```python
from build123d import *

# Parameters (mm, degrees)
EXTRUDE_THIN1_DEPTH = 342.9
CUT_EXTRUDE4_REACH  = 348.468
SKETCH2_R           = 2.667


with BuildPart() as part:
    # Sketch1 → Extrude-Thin1 (new, symmetric)
    with BuildSketch(Plane(origin=(0, 0, 0), x_dir=(0, 0, -1), z_dir=(1, 0, 0))):
        Polygon((-38.1, 0), (0, 0), (0, 38.1), (-6.35, 38.1), (-6.35, 6.35), (-38.1, 6.35), align=None)
    extrude(amount=EXTRUDE_THIN1_DEPTH, both=True)

    # Sketch2 → Cut-Extrude4 (cut, up to next)
    with BuildSketch(Plane(origin=(0, 6.35, 0), x_dir=(1, 0, 0), z_dir=(0, 1, 0)), mode=Mode.PRIVATE) as cut_extrude4_sk1:
        with Locations(Location((-336.55, -15.875, 0), (0, 0, 270))):
            Circle(SKETCH2_R)
    cut_extrude4_tool1 = extrude(cut_extrude4_sk1.sketch, amount=-CUT_EXTRUDE4_REACH, mode=Mode.PRIVATE) & part.part
    # Sketch2 → Cut-Extrude4 (cut, up to next)
    with BuildSketch(Plane(origin=(0, 6.35, 0), x_dir=(1, 0, 0), z_dir=(0, 1, 0)), mode=Mode.PRIVATE) as cut_extrude4_sk2:
        with Locations(Location((-273.05, -15.875, 0), (0, 0, 270))):
            Circle(SKETCH2_R)
    cut_extrude4_tool2 = extrude(cut_extrude4_sk2.sketch, amount=-CUT_EXTRUDE4_REACH, mode=Mode.PRIVATE) & part.part
    # Sketch2 → Cut-Extrude4 (cut, up to next)
    with BuildSketch(Plane(origin=(0, 6.35, 0), x_dir=(1, 0, 0), z_dir=(0, 1, 0)), mode=Mode.PRIVATE) as cut_extrude4_sk3:
        with Locations(Location((-209.55, -15.875, 0), (0, 0, 270))):
            Circle(SKETCH2_R)
    cut_extrude4_tool3 = extrude(cut_extrude4_sk3.sketch, amount=-CUT_EXTRUDE4_REACH, mode=Mode.PRIVATE) & part.part
    # Sketch2 → Cut-Extrude4 (cut, up to next)
    with BuildSketch(Plane(origin=(0, 6.35, 0), x_dir=(1, 0, 0), z_dir=(0, 1, 0)), mode=Mode.PRIVATE) as cut_extrude4_sk4:
        with Locations(Location((-196.85, -15.875, 0), (0, 0, 270))):
            Circle(SKETCH2_R)
    cut_extrude4_tool4 = extrude(cut_extrude4_sk4.sketch, amount=-CUT_EXTRUDE4_REACH, mode=Mode.PRIVATE) & part.part
    # Sketch2 → Cut-Extrude4 (cut, up to next)
    with BuildSketch(Plane(origin=(0, 6.35, 0), x_dir=(1, 0, 0), z_dir=(0, 1, 0)), mode=Mode.PRIVATE) as cut_extrude4_sk5:
        with Locations(Location((-57.15, -15.875, 0), (0, 0, 270))):
            Circle(SKETCH2_R)
    cut_extrude4_tool5 = extrude(cut_extrude4_sk5.sketch, amount=-CUT_EXTRUDE4_REACH, mode=Mode.PRIVATE) & part.part
    # Sketch2 → Cut-Extrude4 (cut, up to next)
    with BuildSketch(Plane(origin=(0, 6.35, 0), x_dir=(1, 0, 0), z_dir=(0, 1, 0)), mode=Mode.PRIVATE) as cut_extrude4_sk6:
        with Locations(Location((-44.45, -15.875, 0), (0, 0, 270))):
            Circle(SKETCH2_R)
    cut_extrude4_tool6 = extrude(cut_extrude4_sk6.sketch, amount=-CUT_EXTRUDE4_REACH, mode=Mode.PRIVATE) & part.part
    # Sketch2 → Cut-Extrude4 (cut, up to next)
    with BuildSketch(Plane(origin=(0, 6.35, 0), x_dir=(1, 0, 0), z_dir=(0, 1, 0)), mode=Mode.PRIVATE) as cut_extrude4_sk7:
        with Locations(Location((44.45, -15.875, 0), (0, 0, 270))):
            Circle(SKETCH2_R)
    cut_extrude4_tool7 = extrude(cut_extrude4_sk7.sketch, amount=-CUT_EXTRUDE4_REACH, mode=Mode.PRIVATE) & part.part
    # Sketch2 → Cut-Extrude4 (cut, up to next)
    with BuildSketch(Plane(origin=(0, 6.35, 0), x_dir=(1, 0, 0), z_dir=(0, 1, 0)), mode=Mode.PRIVATE) as cut_extrude4_sk8:
        with Locations(Location((57.15, -15.875, 0), (0, 0, 270))):
            Circle(SKETCH2_R)
    cut_extrude4_tool8 = extrude(cut_extrude4_sk8.sketch, amount=-CUT_EXTRUDE4_REACH, mode=Mode.PRIVATE) & part.part
    # Sketch2 → Cut-Extrude4 (cut, up to next)
    with BuildSketch(Plane(origin=(0, 6.35, 0), x_dir=(1, 0, 0), z_dir=(0, 1, 0)), mode=Mode.PRIVATE) as cut_extrude4_sk9:
        with Locations(Location((196.85, -15.875, 0), (0, 0, 270))):
            Circle(SKETCH2_R)
    cut_extrude4_tool9 = extrude(cut_extrude4_sk9.sketch, amount=-CUT_EXTRUDE4_REACH, mode=Mode.PRIVATE) & part.part
    # Sketch2 → Cut-Extrude4 (cut, up to next)
    with BuildSketch(Plane(origin=(0, 6.35, 0), x_dir=(1, 0, 0), z_dir=(0, 1, 0)), mode=Mode.PRIVATE) as cut_extrude4_sk10:
        with Locations(Location((209.55, -15.875, 0), (0, 0, 270))):
            Circle(SKETCH2_R)
    cut_extrude4_tool10 = extrude(cut_extrude4_sk10.sketch, amount=-CUT_EXTRUDE4_REACH, mode=Mode.PRIVATE) & part.part
    # Sketch2 → Cut-Extrude4 (cut, up to next)
    with BuildSketch(Plane(origin=(0, 6.35, 0), x_dir=(1, 0, 0), z_dir=(0, 1, 0)), mode=Mode.PRIVATE) as cut_extrude4_sk11:
        with Locations(Location((336.55, -15.875, 0), (0, 0, 270))):
            Circle(SKETCH2_R)
    cut_extrude4_tool11 = extrude(cut_extrude4_sk11.sketch, amount=-CUT_EXTRUDE4_REACH, mode=Mode.PRIVATE) & part.part
    # Sketch2 → Cut-Extrude4 (cut, up to next)
    with BuildSketch(Plane(origin=(0, 6.35, 0), x_dir=(1, 0, 0), z_dir=(0, 1, 0)), mode=Mode.PRIVATE) as cut_extrude4_sk12:
        with Locations(Location((273.05, -15.875, 0), (0, 0, 270))):
            Circle(SKETCH2_R)
    cut_extrude4_tool12 = extrude(cut_extrude4_sk12.sketch, amount=-CUT_EXTRUDE4_REACH, mode=Mode.PRIVATE) & part.part
    add(cut_extrude4_tool1.solids().sort_by_distance((-336.55, 6.35, 15.875))[0], mode=Mode.SUBTRACT)
    add(cut_extrude4_tool2.solids().sort_by_distance((-273.05, 6.35, 15.875))[0], mode=Mode.SUBTRACT)
    add(cut_extrude4_tool3.solids().sort_by_distance((-209.55, 6.35, 15.875))[0], mode=Mode.SUBTRACT)
    add(cut_extrude4_tool4.solids().sort_by_distance((-196.85, 6.35, 15.875))[0], mode=Mode.SUBTRACT)
    add(cut_extrude4_tool5.solids().sort_by_distance((-57.15, 6.35, 15.875))[0], mode=Mode.SUBTRACT)
    add(cut_extrude4_tool6.solids().sort_by_distance((-44.45, 6.35, 15.875))[0], mode=Mode.SUBTRACT)
    add(cut_extrude4_tool7.solids().sort_by_distance((44.45, 6.35, 15.875))[0], mode=Mode.SUBTRACT)
    add(cut_extrude4_tool8.solids().sort_by_distance((57.15, 6.35, 15.875))[0], mode=Mode.SUBTRACT)
    add(cut_extrude4_tool9.solids().sort_by_distance((196.85, 6.35, 15.875))[0], mode=Mode.SUBTRACT)
    add(cut_extrude4_tool10.solids().sort_by_distance((209.55, 6.35, 15.875))[0], mode=Mode.SUBTRACT)
    add(cut_extrude4_tool11.solids().sort_by_distance((336.55, 6.35, 15.875))[0], mode=Mode.SUBTRACT)
    add(cut_extrude4_tool12.solids().sort_by_distance((273.05, 6.35, 15.875))[0], mode=Mode.SUBTRACT)


solid = part.part
```
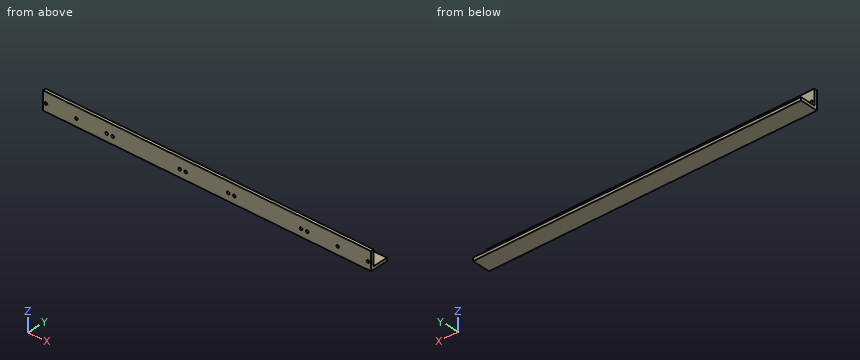
Read the model definition and answer for the solid it produces. Units are mm, in the model's axes. Give positions to 0.01 mm unless a question says otherwise; leave off trailing zeros. Loops run counter-clockwise (first coordinate to the right, second up) from the corner with the lowest first, then second, coordinate; pieces in that order, holes last.
Item 1: Each of these flat-tipped pins is pushed along its axis until it touches: pin 1 Ø7 at (x, z) = (-196.85, 15.875) entering from +Y; pin 2 Ø3 at (x, z) = (-273.05, 15.875) entering from +Y; pin 3 Ø1 at (x, y) = (-257, 7.5) entering from +Z. Where does it stop, or does it pass through?
Item 2: Find the intervals of material crossed by line 1 along Z through (x, y) = (-196.85, 3.5); line 2 along Y through (x, z) = (-9, 11.5), in increasing order.
Item 3: The part is cut by section A-A (x = -123). Write down the section's boundary in (y, z).
Item 4: The part is cut by section B-B (y = 30). Write down the section's boundary in (x, z), and give its area (3 significant figures).
Taken from the geometry:
1. pin 1: stops at y = 6.35
1. pin 2: passes through
1. pin 3: stops at z = 6.35
2. line 1: z = 0 to 13.21, 18.54 to 38.1
2. line 2: y = 0 to 6.35
3. outline: (0, 0) - (38.1, 0) - (38.1, 6.35) - (6.35, 6.35) - (6.35, 38.1) - (0, 38.1) - close
4. outline: (-342.9, 0) - (342.9, 0) - (342.9, 6.35) - (-342.9, 6.35) - close
4. area: 4,350 mm2
